Source: CAD feature listing. Evaluate the final solid. Frame: model axes, mm. A direction names the side the tool comes from. Round coordinates to 2 decimals unless told otherwise and drop trailing zeros. Order: outer loops, then holes, each group sorted by start corner. A loop starts at its lowest first (then second) coordinate and runs counter-clockwise, first axis right, second up. Notation, with made-up numbers: (31, 76) -> (55, 76) arc R30 cw to (55, 104) -> close; hole circle Ø1 at (-25, 59.25). An arc over 180 degrees is marked (long way). One line per item, written item: value. Start each with the question number.
1) Section C-C (y = 1.3). Return the cut outline in (x, z).
2) Section D-D (x = 14.5). Return the cut outline in (y, z).
3) Pin query (flat end, axial travel): P1, Ø4.5, axis at x = 31.75, z = 0, coming from the +Y side; P2, Ø1.5, axis at x = 16.5, y = 3, coming from the -Z side; P3, Ø2, axis at x = -31.75, z = 0, coming from the +Y side. Return the tip coordinate at first contact, or that it passes through.
4) Section A-A (x = 31.75). Return the cut outline in (y, z).
5) Mould query, pull axis X, two halves, no side actions, for faces 3 (the face through (-1, 0, -5)), 4 (the face through (-38, 1, -9)), 5 (the face through (37, 1, -10)), 6 (the face through (-35.25, 2, 0)). Classes: pulls with the +X half, pulls with the -X half, needs draft (parallel to the pull), parting line crosses it, or undercut.
6) Reachability of faces 1 (the face through (0, 0.5, -6)), 2 (the face through (-38.43, 3.4, -0.08)) from +Z, -Z, +X, -X, +Y, -Y: full face, straight path, thin tool, end or side. Return the list, or none.
7) Ray query, L1, parallel to X at y = 0.2, z = 0; L2, parallel to X at y = 0.2, z = 4.5; L3, parallel to Z at x = 34, y = 2.2. Return the intervals inside material, ascending.
8) Section B-B (z = 0). Return the cut outline in (x, y), and give its area (3 significant figures).
```python
from build123d import *
from OCP.BRepFilletAPI import BRepFilletAPI_MakeFillet

# Parameters (mm, degrees)
SKETCH2_W           = 72
SKETCH2_H           = 18
SKETCH2_R           = 1.7
SKETCH2_W_2         = 56.7
SKETCH2_H_2         = 9.5
BOSS_EXTRUDE2_DEPTH = 0.5
SKETCH3_W           = 78
SKETCH3_H           = 22
SKETCH3_W_2         = 70.5
SKETCH3_H_2         = 13.5
BOSS_EXTRUDE3_DEPTH = 4
FILLET1_R1          = 5
FILLET1_R2          = 2


with BuildPart() as part:
    # Sketch2 → Boss-Extrude2 (new body)
    with BuildSketch(Plane(origin=(0, 0, 0), x_dir=(1, 0, 0), z_dir=(0, 1, 0))):
        Rectangle(SKETCH2_W, SKETCH2_H)
        with Locations(Location((-31.75, 0, 0), (0, 0, 270))):
            Circle(SKETCH2_R, mode=Mode.SUBTRACT)
        with Locations(Location((31.75, 0, 0), (0, 0, 270))):
            Circle(SKETCH2_R, mode=Mode.SUBTRACT)
        Rectangle(SKETCH2_W_2, SKETCH2_H_2, mode=Mode.SUBTRACT)
    extrude(amount=BOSS_EXTRUDE2_DEPTH)

    # Sketch3 → Boss-Extrude3 (add)
    with BuildSketch(Plane(origin=(0, 0, 0), x_dir=(1, 0, 0), z_dir=(0, 1, 0))):
        Rectangle(SKETCH3_W, SKETCH3_H)
        Rectangle(SKETCH3_W_2, SKETCH3_H_2, mode=Mode.SUBTRACT)
    extrude(amount=BOSS_EXTRUDE3_DEPTH)

    # Fillet1: one fillet with a radius per group of edges: ONE call of the kernel's fillet builder (fillet() takes one radius for all edges)
    fillet1_edges_1 = [part.edges().sort_by_distance(p)[0] for p in [
        (-39, 2, -11),
        (-39, 2, 11),
        (39, 2, 11),
        (39, 2, -11),
    ]]
    fillet1_edges_2 = [part.edges().sort_by_distance(p)[0] for p in [
        (0, 4, -11),
        (-39, 4, 0),
        (0, 4, 11),
        (39, 4, 0),
    ]]
    fillet1 = BRepFilletAPI_MakeFillet(part.part.solid().wrapped)
    for e in fillet1_edges_1:
        fillet1.Add(FILLET1_R1, e.wrapped)
    for e in fillet1_edges_2:
        fillet1.Add(FILLET1_R2, e.wrapped)
    add(Compound.cast(fillet1.Shape()), mode=Mode.REPLACE)


solid = part.part
```
Findings:
1. outline: (-39, -6) arc R5 ccw to (-34, -11) -> (34, -11) arc R5 ccw to (39, -6) -> (39, 6) arc R5 ccw to (34, 11) -> (-34, 11) arc R5 ccw to (-39, 6) -> close; hole (-35.25, -6.75) -> (35.25, -6.75) -> (35.25, 6.75) -> (-35.25, 6.75) -> close
2. outline: (0, -11) -> (2, -11) arc R2 ccw to (4, -9) -> (4, -6.75) -> (0.5, -6.75) -> (0.5, -4.75) -> (0, -4.75) -> close; (0, 4.75) -> (0.5, 4.75) -> (0.5, 6.75) -> (4, 6.75) -> (4, 9) arc R2 ccw to (2, 11) -> (0, 11) -> close
3. P1: y = 0.5
3. P2: z = -10.98
3. P3: through
4. outline: (0, -11) -> (2, -11) arc R2 ccw to (4, -9) -> (4, -6.75) -> (0.5, -6.75) -> (0.5, -1.7) -> (0, -1.7) -> close; (0, 1.7) -> (0.5, 1.7) -> (0.5, 6.75) -> (4, 6.75) -> (4, 9) arc R2 ccw to (2, 11) -> (0, 11) -> close
5. face 3: needs draft
5. face 4: pulls with the -X half
5. face 5: pulls with the +X half
5. face 6: undercut
6. face 1: +Y
6. face 2: +Z, -Z, -X, +Y
7. L1: -39 to -33.45, -30.05 to -28.35, 28.35 to 30.05, 33.45 to 39
7. L2: -39 to -28.35, 28.35 to 39
7. L3: -10.99 to -6.75, 6.75 to 10.99
8. outline: (-39, 0) -> (-33.45, 0) -> (-33.45, 0.5) -> (-35.25, 0.5) -> (-35.25, 4) -> (-37, 4) arc R2 ccw to (-39, 2) -> close; (-30.05, 0) -> (-28.35, 0) -> (-28.35, 0.5) -> (-30.05, 0.5) -> close; (28.35, 0) -> (30.05, 0) -> (30.05, 0.5) -> (28.35, 0.5) -> close; (33.45, 0) -> (39, 0) -> (39, 2) arc R2 ccw to (37, 4) -> (35.25, 4) -> (35.25, 0.5) -> (33.45, 0.5) -> close
8. area: 31.8 mm2
